Source: CAD feature listing. Evaluate the final solid. Frame: model axes, mm. A direction names the side the tool comes from. Round coordinates to 2 decimals unless told otherwise and drop trailing zeros. Loops run counter-clockwise (first coordinate to the right, second up) from the corner with the lowest first, then second, coordinate; pieces in that order, holes last. Notation, with made-up numbers: (-3, 17.5) -> (46, 17.5) arc R27 cw to (46, 37.5) -> close; hole circle Ø2 at (88, -36). An arc over 180 degrees is marked (long way). Write item = value, one per line.
from build123d import *

# Parameters (mm, degrees)
F3_DEPTH  = 172
F4_DEPTH  = 150
F7_DEPTH  = 111
F8_DEPTH  = 163
F10_DEPTH = 42
F11_DEPTH = 89
F14_DEPTH = 110
F17_W     = 21
F17_H     = 53
F18_DEPTH = 21
F1_W      = 23
F1_H      = 42
F19_DEPTH = 18


with BuildPart() as f3:
    # F0 (on Front) → F3 (new body)
    with BuildSketch(Plane.XZ):
        Polygon((0, 92), (0, 0), (75, 0), (75, 28.440581), (63.021571, 53), (44, 92), align=None)
    extrude(amount=-F3_DEPTH)

    # F2 (on Right) → F4 (intersect)
    with BuildSketch(Plane.YZ):
        Polygon((0, 67), (0, 0), (121, 0), (121, 53), (106.029303, 92), (25, 92), align=None)
    extrude(amount=F4_DEPTH, mode=Mode.INTERSECT)


with BuildPart() as f7:
    # F6 (on offset) → F7 (new body)
    with BuildSketch(Plane.XZ.offset(-44)):
        Polygon((0, 92), (0, 0), (110, 0), (110, 53), (71, 92), align=None)
    extrude(amount=-F7_DEPTH)


with BuildPart() as f8_tool:
    # F2 (on Right) → F8 (new body)
    with BuildSketch(Plane.YZ):
        Polygon((0, 67), (0, 0), (121, 0), (121, 53), (106.029303, 92), (25, 92), align=None)
    extrude(amount=F8_DEPTH)


with BuildPart() as f3_1:
    add(f3.part)

    # F8: intersect by f8_tool
    add(f8_tool.part, mode=Mode.INTERSECT)

    # F9 (on face) → F10 (cut)
    with BuildSketch(Plane.YZ.offset(75)):
        with BuildLine():
            Line((0, 0), (44, 0))
            ThreePointArc((44, 0), (41.311037, 15.145899), (33.572807, 28.440581))
            Line((33.572807, 28.440581), (0, 28.440581))
            Line((0, 28.440581), (0, 0))
        make_face()
        with BuildLine():
            ThreePointArc((33.572807, 28.440581), (-41.311037, -15.145899), (44, 0))
            Line((44, 0), (0, 0))
            Line((0, 0), (0, 28.440581))
            Line((0, 28.440581), (33.572807, 28.440581))
        make_face()
    extrude(amount=-F10_DEPTH, mode=Mode.SUBTRACT)


with BuildPart() as f7_1:
    add(f7.part)

    # F8: intersect by f8_tool
    add(f8_tool.part, mode=Mode.INTERSECT)


with BuildPart() as f11:
    # F0 (on Front) → F11 (new body)
    with BuildSketch(Plane.XZ):
        Polygon((113.488927, 92), (44, 92), (63.021571, 53), (113.488927, 53), align=None)
    extrude(amount=-F11_DEPTH)


with BuildPart() as f7_2:
    add(f7_1.part)

    # F12: cut F11
    add(f11.part, mode=Mode.SUBTRACT)


with BuildPart() as f14:
    # F13 (on face) → F14 (new body)
    with BuildSketch(Plane.YZ.offset(110)):
        Polygon((44, 53), (44, 0), (60.203726, 53), align=None)
    extrude(amount=-F14_DEPTH)


with BuildPart() as f7_3:
    add(f7_2.part)

    # F15: cut F14
    add(f14.part, mode=Mode.SUBTRACT)


with BuildPart() as f3_2:
    add(f3_1.part)

    # F16: union F7
    add(f7_3.part)

    # F17 (on face) → F18 (cut)
    with BuildSketch(Plane.XY.offset(92)):
        with Locations((33.5, 62.5)):
            Rectangle(F17_W, F17_H)
        Polygon((71, 89), (44, 89), (44, 36), (84.379675, 36), (84.379675, 89), align=None)
    extrude(amount=-F18_DEPTH, mode=Mode.SUBTRACT)

    # F1 (on Top) → F19 (cut)
    with BuildSketch(Plane.XY):
        with Locations((11.5, 100)):
            Rectangle(F1_W, F1_H)
    extrude(amount=F19_DEPTH, mode=Mode.SUBTRACT)


solid = f3_2.part
1. Section query A-A (x = 42). Return the cut outline in (y, z).
Evaluation:
outline = (0, 44) arc R44 cw to (33.57, 28.44) arc R44 cw to (44, 0) -> (121, 0) -> (121, 53) -> (106.03, 92) -> (89, 92) -> (89, 71) -> (36, 71) -> (36, 92) -> (25, 92) -> (0, 67) -> close
2. Line query: probe 1 along X at (y, z) = (53, 83); probe 2 along Z at (x, y) = (5, 84.5); probe 3 along Z at (x, y) = (45.5, 82). Output: solid intervals per line, ascending. Write a range as from..to.
Evaluation:
probe_1 = 0..23
probe_2 = 18..92
probe_3 = 0..71
3. Section query D-D (y = 98.5). Return the cut outline in (x, z), then the cut area to 3 significant figures.
Evaluation:
outline = (0, 18) -> (23, 18) -> (23, 0) -> (110, 0) -> (110, 53) -> (71, 92) -> (0, 92) -> close
area = 8,950 mm²
4. Contact query for flat-ended pins moving along their axis: pin 1 Ø20 at (x, z) = (12.5, 6.5) entering from +Y; pin 2 Ø11.5 at (x, z) = (86.5, 78) entering from -Y; pin 3 Ø2 at (y, z) = (51, 37) entering from -X; pin 4 Ø4 at (x, y) = (36, 18.5) entering from -Z. Output: stop coordinate, or through.
Evaluation:
pin_1 = 79
pin_2 = 89
pin_3 = 0
pin_4 = 38.93
5. Mould query, pull axis Y, two halves, no side actions, for faces 6 (the face through (66, 89, 73)), 7 (the face through (28, 13, 80)), 8 (the face through (75, 45, 20)). Classes: released by +Y, released by -Y, zero draft, split by the parting line, or undercut.
Evaluation:
face_6 = undercut
face_7 = released by -Y
face_8 = zero draft
6. Section query B-B (y = 68). Return the cut outline in (x, z), then the cut area to 3 significant figures.
Evaluation:
outline = (0, 0) -> (110, 0) -> (110, 53) -> (63.02, 53) -> (54.24, 71) -> (23, 71) -> (23, 92) -> (0, 92) -> close
area = 7,370 mm²
7. Set-up query: faces 1 (the face through (23, 100, 9)), 2 (the face through (38, 63, 71)), 3 (the face through (92.06, 51.99, 26.13)), 4 (the face through (33, 17, 17)), 5 (the face through (110, 82, 26)). Return all of +Z, -Z, +X, -X, +Y, -Y with unobstructed straight access to the full face (end or side cutting, diameter ignored); none if empty.
Evaluation:
face_1 = -Z, -X, +Y
face_2 = +Z, +X
face_3 = +Z, +X, -Y
face_4 = -Z, +X, -Y
face_5 = +Z, -Z, +X, +Y, -Y
8. Section query C-C (z = 83). Return the cut outline in (x, y).
Evaluation:
outline = (0, 16) -> (48.39, 16) -> (48.39, 36) -> (23, 36) -> (23, 89) -> (80, 89) -> (80, 109.48) -> (0, 109.48) -> close
